```python
from build123d import *

# Parameters (mm, degrees)
SKETCH1_R           = 11
SKETCH1_W           = 28.025444105
SKETCH1_H           = 13.338271477
BOSS_EXTRUDE1_DEPTH = 2
SKETCH2_W           = 28.025444105
SKETCH2_H           = 13.338271477
BOSS_EXTRUDE2_DEPTH = 1


with BuildPart() as part:
    # Sketch1 → Boss-Extrude1 (new body)
    with BuildSketch(Plane.XY):
        with BuildLine():
            Line((420.808310711, 971.794452341), (420.808310711, 1008.244630448))
            Line((420.808310711, 1008.244630448), (452.024309123, 1008.244630448))
            Line((452.024309123, 1008.244630448), (452.024309123, 971.794452341))
            ThreePointArc((452.024309123, 971.794452341), (436.416309917, 956.186453136), (420.808310711, 971.794452341))
        make_face()
        with Locations((436.416309917, 971.794452341)):
            Circle(SKETCH1_R, mode=Mode.SUBTRACT)
        with Locations((436.489180342, 1000.019726734)):
            Rectangle(SKETCH1_W, SKETCH1_H, mode=Mode.SUBTRACT)
    extrude(amount=BOSS_EXTRUDE1_DEPTH)

    # Sketch2 → Boss-Extrude2 (add)
    with BuildSketch(Plane.XY):
        with Locations((436.489180342, 1000.019726734)):
            Rectangle(SKETCH2_W, SKETCH2_H)
    extrude(amount=BOSS_EXTRUDE2_DEPTH)


solid = part.part
```
The model under review builds one solid part; all positions refer to its coordinate system, in mm. A direction names the side the tool comes from. Give positions to 0.01 mm unless a question says otherwise; leave off trailing zeros. Write each loop counter-clockwise with the first axis right and the second up, starting at its lowest first coordinate (ties: lowest second). Pieces come first, ordered by that corner, then holes. Notation, with made-up numbers: (26, 16.5) - (41, 16.5) arc R26 ccw to (41, 48.5) - close; hole circle Ø2 at (-16, -3). An arc over 180 degrees is marked (long way). Answer in a Markdown table with one row per item. Add a question column.
1. We need section C-C on y = 965. Write out the cut boundary in (x, z).
2. We need section D-D on y = 1002. Write out the cut boundary in (x, z).
3. Insertion check: P1, Ø6.5, axis at x = 430, y = 998.5, coming from the +Z side; P2, Ø1.1, axis at x = 430.5, z = 1.5, coming from the -Y side; P3, Ø6, axis at x = 439, y = 1001, coming from the -Z side; P4, Ø17.5, axis at x = 436.42, y = 971.79, coming from the -Z side. Each pin has a flat end and moves straight along its axis. Give the tip position at first contact, or say it passes through.
4. Wall thickness on line 1 along Y through (x, z) = (436.5, 1.9); line 2 along Y through (x, z) = (429, 1.3); line 3 along X through (y, z) = (973.5, 1.05): over which ranges is each line inside the solid? List them lowest first. Write a range as [from, to].
5. Tool access review of faces 1 (the flat face through (440, 983, 2)), 2 (the flat face through (436, 1000, 1)): name each direction out of +Z, -Z, +X, -X, +Y, -Y from which nothing blocks a thin tool from reaching the whole face with its end or side.
6. Draft analysis for pull direction Y (two halves, no side actions). For faces 3 (the cylindrical face through (434.98, 982.7, 0.99)), 4 (the flat face through (436, 1008.245, 1)), 5 (the cylindrical face through (436.76, 956.19, 0.99)), 6 (the flat face through (436, 988, 0)), state which applies: +Y half, -Y half, draft (parallel to the pull), parting line (faces both ways), or undercut.
7. We need section B-B on x = 426. Write out the cut boundary in (y, z), then the cut area to 3 significant figures.
Ans:
| question | item | result |
|---|---|---|
| 1 | outline | (422.36, 0) - (427.77, 0) - (427.77, 2) - (422.36, 2) - close; (445.07, 0) - (450.47, 0) - (450.47, 2) - (445.07, 2) - close |
| 2 | outline | (420.81, 0) - (452.02, 0) - (452.02, 2) - (450.5, 2) - (450.5, 1) - (422.48, 1) - (422.48, 2) - (420.81, 2) - close |
| 3 | P1 | stops at z = 1 |
| 3 | P2 | stops at y = 957.14 |
| 3 | P3 | stops at z = 0 |
| 3 | P4 | passes through |
| 4 | line 1 | y = [956.19, 960.79], [982.79, 993.35], [1006.69, 1008.24] |
| 4 | line 2 | y = [958.06, 963.67], [979.92, 993.35], [1006.69, 1008.24] |
| 4 | line 3 | x = [420.81, 425.55], [447.28, 452.02] |
| 5 | face 1 | +Z, +X, -X, +Y, -Y |
| 5 | face 2 | +Z |
| 6 | face 3 | undercut |
| 6 | face 4 | +Y half |
| 6 | face 5 | -Y half |
| 6 | face 6 | draft |
| 7 | outline | (960.17, 0) - (968.26, 0) - (968.26, 2) - (960.17, 2) - close; (975.33, 0) - (1008.24, 0) - (1008.24, 2) - (1006.69, 2) - (1006.69, 1) - (993.35, 1) - (993.35, 2) - (975.33, 2) - close |
| 7 | area | 68.7 mm^2 |
